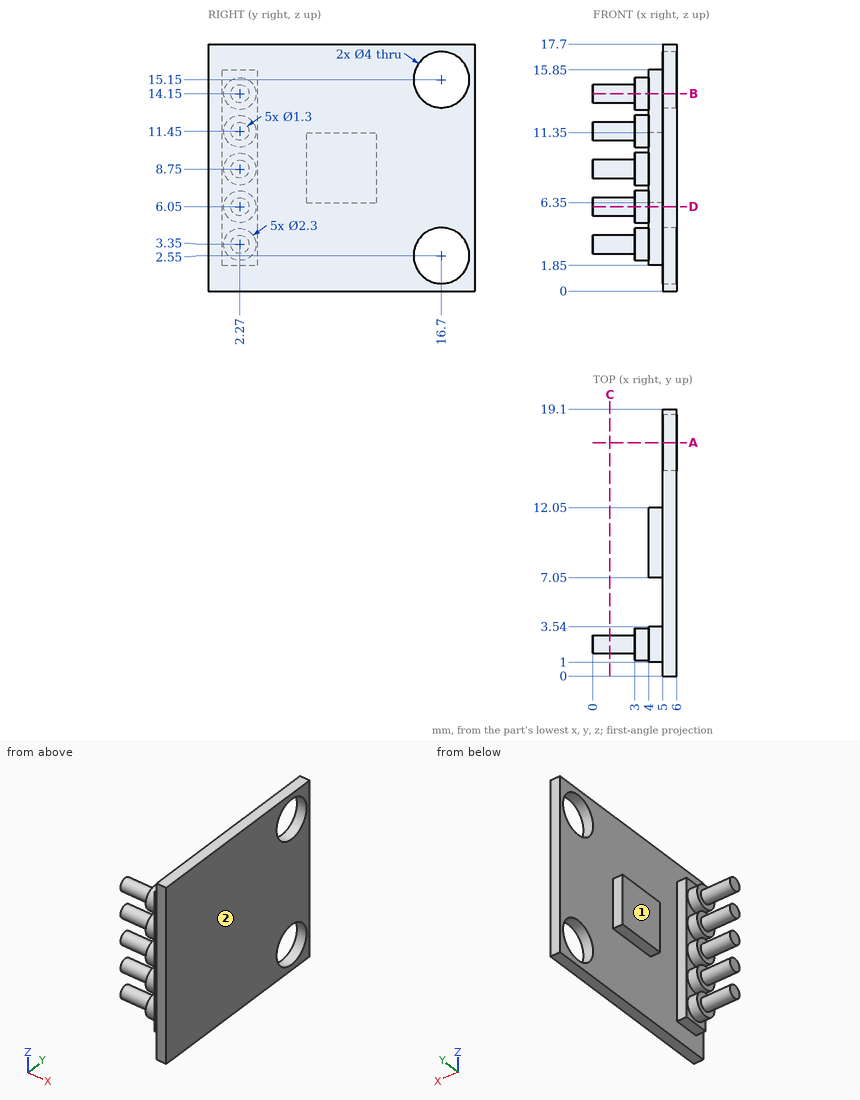
Verification items for this drawing (mm, ordinates from the low corner). A direction names the side the tool comes from. Give positions to 0.01 mm unless a question says otherwise; leave off trailing zeros. Loops run counter-clockwise (first coordinate to the right, second up) from the corner with the lowest first, then second, coordinate; pieces in that order, holes last.
1. Cross-section at B-B on z = 14.15. Record the cut outline in (x, y), and give its area (3 significant figures).
Derived:
outline: (0, 1.62) - (3, 1.62) - (3, 1.12) - (4, 1.12) - (4, 1) - (5, 1) - (5, 0) - (6, 0) - (6, 14.97) - (5, 14.97) - (5, 3.54) - (4, 3.54) - (4, 3.42) - (3, 3.42) - (3, 2.92) - (0, 2.92) - close; (5, 18.43) - (6, 18.43) - (6, 19.1) - (5, 19.1) - close
area: 24.4 mm2
2. Material ranges on probe 1 along Y at (x, z) = (5.75, 2.55); probe 2 along Z at (x, y) = (2.65, 2.25); probe 3 along Y at (x, z) = (4.45, 10), recorded low to high.
Derived:
probe 1: y = 0 to 14.7, 18.7 to 19.1
probe 2: z = 2.7 to 4, 5.4 to 6.7, 8.1 to 9.4, 10.8 to 12.1, 13.5 to 14.8
probe 3: y = 1 to 3.54, 7.05 to 12.05
3. Cross-section at A-A on y = 16.7. Record the cut outline in (x, z), and give its area (3 significant figures).
Derived:
outline: (5, 0) - (6, 0) - (6, 0.55) - (5, 0.55) - close; (5, 4.55) - (6, 4.55) - (6, 13.15) - (5, 13.15) - close; (5, 17.15) - (6, 17.15) - (6, 17.7) - (5, 17.7) - close
area: 9.70 mm2
4. Go/stop test with flat-tipped pins: P1, Ø2.5, axis at y = 1.5, z = 8.5, coming from the -X side; P2, Ø0.8, axis at x = 4.5, y = 9.5, coming from the +Z side; P3, Ø1, axis at y = 6.5, z = 11, coming from the -X side; P4, Ø0.8, axis at x = 4.5, z = 5.5, coming from the -Y side. Record where each tip stops, or that it passes through.
Derived:
P1: stops at x = 0
P2: stops at z = 11.35
P3: stops at x = 5
P4: stops at y = 1
5. Cross-section at D-D on z = 6.05. Record the cut outline in (x, y).
Derived:
outline: (0, 1.62) - (3, 1.62) - (3, 1.12) - (4, 1.12) - (4, 1) - (5, 1) - (5, 0) - (6, 0) - (6, 19.1) - (5, 19.1) - (5, 3.54) - (4, 3.54) - (4, 3.42) - (3, 3.42) - (3, 2.92) - (0, 2.92) - close
6. Cross-section at C-C on x = 1.2. Record the cut outline in (y, z).
Derived:
outline: circle Ø1.3 at (2.27, 3.35); circle Ø1.3 at (2.27, 6.05); circle Ø1.3 at (2.27, 8.75); circle Ø1.3 at (2.27, 11.45); circle Ø1.3 at (2.27, 14.15)
7. Tool access check on the marked faces 1 and 2. Record the directions out of +Z, -Z, +X, -X, +Y, -Y that give a thin tool (end or side, any length) a straight path to the whole face; none if there is none.
Derived:
face 1: +Z, -Z, -X, +Y
face 2: +Z, -Z, +X, +Y, -Y
